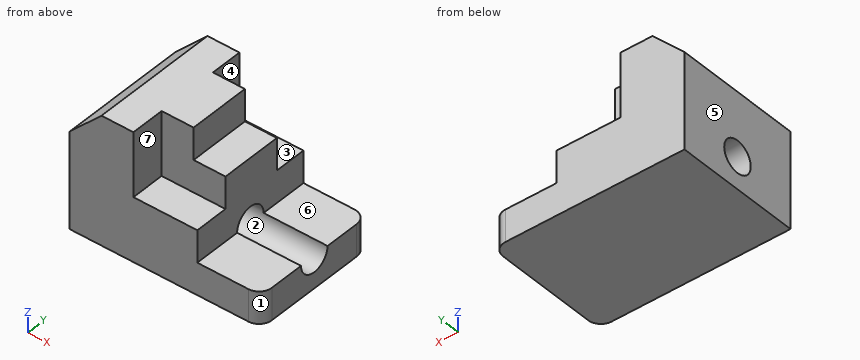
from build123d import *

# Parameters (mm, degrees)
F1_DEPTH = 25.4
F2_W     = 12.7
F2_H     = 12.7
F2_H_2   = 13.5122093648
F3_DEPTH = 25.4
F4_R     = 6.35
F5_DEPTH = 76.201
F6_R     = 5.08


with BuildPart() as f1:
    # F0 (on Front) → F1 (new body, symmetric)
    with BuildSketch(Plane.XZ):
        Polygon((0, 38.1), (0, 0), (76.2, 0), (76.2, 12.7), (50.8, 12.7), (50.8, 25.4), (25.4, 25.4), (25.4, 50.8), (12.7, 50.8), align=None)
        Polygon((38.1, 50.8), (25.4, 50.8), (25.4, 25.4), (50.8, 25.4), (50.8, 38.1), (38.1, 38.1), align=None)
    extrude(amount=F1_DEPTH, both=True)

    # F2 (on face) → F3 (cut)
    with BuildSketch(Plane.XY.offset(50.8)):
        with Locations((44.45, 19.05)):
            Rectangle(F2_W, F2_H)
        with Locations((31.75, 19.05)):
            Rectangle(F2_W, F2_H)
        with Locations((31.75, -18.6438953176)):
            Rectangle(F2_W, F2_H_2)
        with Locations((44.45, -18.6438953176)):
            Rectangle(F2_W, F2_H_2)
    extrude(amount=-F3_DEPTH, mode=Mode.SUBTRACT)

    # F4 (on Right) → F5 (cut, through all)
    with BuildSketch(Plane.YZ):
        with Locations((0, 12.7)):
            Circle(F4_R)
    extrude(amount=F5_DEPTH, mode=Mode.SUBTRACT)

    # F6
    f6_edges = [f1.edges().sort_by_distance(p)[0] for p in [
        (76.2, -25.4, 6.35),
        (76.2, 25.4, 6.35),
    ]]
    fillet(f6_edges, radius=F6_R)


solid = f1.part
Source: CAD feature listing. Evaluate the final solid. Frame: model axes, mm. Face numbers are marked on the shaded views. A direction names the side the tool comes from. Round coordinates to 2 decimals unless told otherwise and drop trailing zeros. Loops run counter-clockwise (first coordinate to the right, second up) from the corner with the lowest first, then second, coordinate; pieces in that order, holes last. Notation, with made-up numbers: (66, -27) -> (121, -27) arc R11 ccw to (121, -21) -> close; hole circle Ø5 at (-23.5, 45.25). An arc over 180 degrees is marked (long way). Answer as a JSON object with one key per item and string values. Group by question number.
Q1. Section query A-A (y = 0). Output: boundary loops of the cut face in (x, z), plus the area to 3 significant figures.
Q2. Mould query, pull axis Y, two halves, no side actions, for the marked faces 1, 2 and 3. Classes: pulls with the +Y half, pulls with the -Y half, needs draft (parallel to the pull), parting line crosses it, or undercut.
Q3. Access query for the marked faces 4, 5, 6 and 7. Directions: +Z, -Z, +X, -X, +Y, -Y. A direction counts if a zero-diameter tool reaches every point of the face in a straight line with its end or side. Return the directions, or none.
Q4. Section query B-B (x = 37). Output: boundary loops of the cut face in (y, z).
Q5. Contact query for flat-ended pins moving along their axis: P1, Ø15, axis at x = 59, y = -19.5, coming from the +Z side; P2, Ø7.5, axis at x = 43.5, z = 40.5, coming from the +Y side; P3, Ø4, axis at y = 18, z = 43, coming from the +X side. Output: stop coordinate, or through.
Q6. Section query D-D (y = -19). Output: boundary loops of the cut face in (x, z).
Q7. Section query C-C (z = 16.5). Output: boundary loops of the cut face in (x, y).
Q8. Ray query, line 1 (Y direction, x = 48.5, z = 12.7); line 2 (X direction, y = -2, z = 32); line 3 (X direction, y = 22, z = 33). Return the intervals inside material, ascending. Write a range as from..to.
Completed:
{
 "1": {"outline": "(0, 0) -> (76.2, 0) -> (76.2, 6.35) -> (0, 6.35) -> close; (0, 19.05) -> (50.8, 19.05) -> (50.8, 38.1) -> (38.1, 38.1) -> (38.1, 50.8) -> (12.7, 50.8) -> (0, 38.1) -> close", "area": "1,850 mm²"},
 "2": {"face 1": "pulls with the -Y half", "face 2": "undercut", "face 3": "needs draft"},
 "3": {"face 4": "+Z, +X, +Y", "face 5": "+Z, -Z, -X, +Y, -Y", "face 6": "+Z, +X, +Y, -Y", "face 7": "+Z, +X, -Y"},
 "4": {"outline": "(-25.4, 0) -> (25.4, 0) -> (25.4, 25.4) -> (12.7, 25.4) -> (12.7, 50.8) -> (-11.89, 50.8) -> (-11.89, 25.4) -> (-25.4, 25.4) -> close; hole circle Ø12.7 at (0, 12.7)"},
 "5": {"P1": "z = 12.7", "P2": "y = 12.7", "P3": "x = 25.4"},
 "6": {"outline": "(0, 0) -> (76.2, 0) -> (76.2, 12.7) -> (50.8, 12.7) -> (50.8, 25.4) -> (25.4, 25.4) -> (25.4, 50.8) -> (12.7, 50.8) -> (0, 38.1) -> close"},
 "7": {"outline": "(0, -25.4) -> (50.8, -25.4) -> (50.8, -5.09) -> (0, -5.09) -> close; (0, 5.09) -> (50.8, 5.09) -> (50.8, 25.4) -> (0, 25.4) -> close"},
 "8": {"line 1": "-25.4..-6.35, 6.35..25.4", "line 2": "0..50.8", "line 3": "0..25.4"}
}
